from build123d import *

# Parameters (mm, degrees)
BOSS_EXTRU_4_DEPTH      = 90
ESQUISSE8_R             = 1.75
ENL_V_MAT_EXTRU_5_DEPTH = 104.440804328
ESQUISSE9_R             = 2.4
ENL_V_MAT_EXTRU_6_DEPTH = 104.440804328
CONG_7_SIZE             = 10
ENL_V_START             = -1.2
ESQUISSE10_R            = 2.25
ESQUISSE10_R_2          = 1.75
ENL_V_MAT_EXTRU_7_DEPTH = 103.240804328


with BuildPart() as part:
    # Esquisse7 → Boss.-Extru.4 (new body)
    with BuildSketch(Plane.XY):
        Polygon((0, 0), (10, 0), (10, 3), (1.2, 3), (1.2, 50), (0, 50), align=None)
    extrude(amount=BOSS_EXTRU_4_DEPTH)

    # Esquisse8 → Enlèv. mat.-Extru.5 (cut, through all)
    with BuildSketch(Plane.ZY):
        with Locations((10.25, 42.75)):
            Circle(ESQUISSE8_R)
        with Locations((10.25, 7.25)):
            Circle(ESQUISSE8_R)
        with Locations((79.75, 7.25)):
            Circle(ESQUISSE8_R)
        with Locations((79.75, 42.75)):
            Circle(ESQUISSE8_R)
    extrude(amount=-ENL_V_MAT_EXTRU_5_DEPTH, mode=Mode.SUBTRACT)

    # Esquisse9 → Enlèv. mat.-Extru.6 (cut, through all)
    with BuildSketch(Plane.XZ):
        with Locations(Location((5.5, 85, 0), (0, 0, 270))):
            Circle(ESQUISSE9_R)
        with Locations(Location((5.5, 5, 0), (0, 0, 270))):
            Circle(ESQUISSE9_R)
    extrude(amount=-ENL_V_MAT_EXTRU_6_DEPTH, mode=Mode.SUBTRACT)

    # Congé7
    # the kernel refuses this chamfer: 10 mm, written as the material it adds along each edge
    with BuildSketch(Plane(origin=(1.2, 3, 0), x_dir=(0.9996219169112968, -0.02749587661058636, 0), z_dir=(0, 0, 1))) as cong_7_piece_1_section:
        Polygon((CONG_7_SIZE * 0.999621916911, CONG_7_SIZE * 0.0274958766106), (-CONG_7_SIZE * 0.0274958766106, CONG_7_SIZE * 0.999621916911), (0, 0), align=None)
    cong_7_piece_1 = extrude(amount=90, mode=Mode.PRIVATE)
    cong_7_piece_1 = split(cong_7_piece_1, bisect_by=Plane(origin=(10, 6.380086708, 44.999999953), z_dir=(-1, 0, 0)), keep=Keep.TOP, mode=Mode.PRIVATE)
    cong_7_piece_1 = cong_7_piece_1 - Plane(origin=(5.5, 6.380086708, 85), x_dir=(0, 0, -1), z_dir=(0, -1, 0)) * Cylinder(2.4, 220, mode=Mode.PRIVATE)
    cong_7_piece_1 = cong_7_piece_1 - Plane(origin=(5.5, 6.380086708, 5), x_dir=(0, 0, -1), z_dir=(0, -1, 0)) * Cylinder(2.4, 220, mode=Mode.PRIVATE)
    cong_7_piece_1 = cong_7_piece_1 - Plane(origin=(4.314878847, 7.25, 79.75), x_dir=(0, 0, 1), z_dir=(-1, 0, 0)) * Cylinder(1.75, 220, mode=Mode.PRIVATE)
    cong_7_piece_1 = cong_7_piece_1 - Plane(origin=(4.314878847, 7.25, 10.25), x_dir=(0, 0, 1), z_dir=(-1, 0, 0)) * Cylinder(1.75, 220, mode=Mode.PRIVATE)
    add(cong_7_piece_1)

    # Esquisse10 → Enlèv. mat.-Extru.7 (cut, through all)
    # profile 1 of 2: a face of its own
    with BuildSketch(Plane.ZY.offset(ENL_V_START)):
        with Locations((10.25, 7.25)):
            Circle(ESQUISSE10_R)
        with Locations((10.25, 7.25)):
            Circle(ESQUISSE10_R_2, mode=Mode.SUBTRACT)
    # profile 2 of 2: a face of its own
    with BuildSketch(Plane.ZY.offset(ENL_V_START)):
        with Locations((79.75, 7.25)):
            Circle(ESQUISSE10_R)
        with Locations((79.75, 7.25)):
            Circle(ESQUISSE10_R_2, mode=Mode.SUBTRACT)
    extrude(amount=-ENL_V_MAT_EXTRU_7_DEPTH, mode=Mode.SUBTRACT)


solid = part.part
Model file for the job. Use its own axes, mm. A direction names the side the tool comes from. Give positions to 0.01 mm unless a question says otherwise; leave off trailing zeros. Loops run counter-clockwise (first coordinate to the right, second up) from the corner with the lowest first, then second, coordinate; pieces in that order, holes last. Notation, with made-up numbers: (16.25, 0.5) -> (29.25, 0.5) arc R8 ccw to (29.25, 5.5) -> close; hole circle Ø6 at (10, 64). An arc over 180 degrees is marked (long way). Use a Markdown table: item, result. Add a question column.
(1) Wall check: line 1 along Y through (x, z) = (0.35, 79.75); line 2 along X through (y, z) = (2.5, 5); line 3 along X through (y, z) = (35, 64). Give the ranges that are in metal, low to high.
(2) Tool access for faces 1 (the cylindrical face through (0.59, 41.04, 9.87)), 2 (the flat face through (1.2, 31, 44)), 3 (the cylindrical face through (4.276, 5.054, 9.762)): list every direction of +Z, -Z, +X, -X, +Y, -Y with a clear straight run to the whole face (end or side of a thin tool).
(3) Slice it at B-B on z = 79.75. List the corners of the cut face in (x, y), and give its area (3 significant figures).
(4) Slice it at D-D on y = 25. List the corners of the cut face in (x, z).
(5) Mould opens along Z. For faces 4 (the flat face through (5.7, 8.5, 44.4)), 5 (the cylindrical face through (3.157, 4.261, 5.52)), 6 (the flat face through (1, 12, 90)) say: +Z half, -Z half, draft (parallel to the pull), parting line (faces both ways), or undercut.
(6) Slice it at A-A on y = 42.75. List the corners of the cut face in (x, z).
(7) Drop flat-ended pins along their axis: pin 1 Ø3 at (y, z) = (7.25, 79.75) entering from -X; pin 2 Ø3.5 at (y, z) = (6.5, 79.5) entering from +X; pin 3 Ø2 at (y, z) = (29.5, 59.5) entering from -X; pin 4 Ø5 at (x, z) = (7.5, 54) entering from +Y. Give the stop position or say it passes through.
(8) Slice it at C-C on x = 5.5. List the corners of the cut face in (y, z).
Filled sheet:
| question | item | result |
|---|---|---|
| 1 | line 1 | 0 to 5.5, 9 to 41, 44.5 to 50 |
| 1 | line 2 | 0 to 3.1, 7.9 to 10 |
| 1 | line 3 | 0 to 1.2 |
| 2 | face 1 | +X, -X |
| 2 | face 2 | +Z, -Z, +X, +Y |
| 2 | face 3 | +X |
| 3 | outline | (0, 0) -> (10, 0) -> (10, 4.2) -> (9.2, 5) -> (1.2, 5) -> (1.2, 5.5) -> (0, 5.5) -> close; (0, 9) -> (1.2, 9) -> (1.2, 9.5) -> (4.7, 9.5) -> (1.2, 13) -> (1.2, 41) -> (0, 41) -> close; (0, 44.5) -> (1.2, 44.5) -> (1.2, 50) -> (0, 50) -> close |
| 3 | area | 101 mm2 |
| 4 | outline | (0, 0) -> (1.2, 0) -> (1.2, 90) -> (0, 90) -> close |
| 5 | face 4 | draft |
| 5 | face 5 | undercut |
| 5 | face 6 | +Z half |
| 6 | outline | (0, 0) -> (1.2, 0) -> (1.2, 8.5) -> (0, 8.5) -> close; (0, 12) -> (1.2, 12) -> (1.2, 78) -> (0, 78) -> close; (0, 81.5) -> (1.2, 81.5) -> (1.2, 90) -> (0, 90) -> close |
| 7 | pin 1 | through |
| 7 | pin 2 | x = 9.45 |
| 7 | pin 3 | x = 0 |
| 7 | pin 4 | y = 9.2 |
| 8 | outline | (0, 0) -> (8.7, 0) -> (8.7, 2.6) -> (0, 2.6) -> close; (0, 7.4) -> (8.7, 7.4) -> (8.7, 8.53) arc R2.25 cw (long way) to (8.7, 11.97) -> (8.7, 78.03) arc R2.25 cw (long way) to (8.7, 81.47) -> (8.7, 82.6) -> (0, 82.6) -> close; (0, 87.4) -> (8.7, 87.4) -> (8.7, 90) -> (0, 90) -> close |
